Here's how the part is built. I have some questions about the finished solid (model axes, mm). Face numbers are marked on the shaded views. Round coordinates to 2 decimals unless told otherwise and drop trailing zeros. Loops run counter-clockwise (first coordinate to the right, second up) from the corner with the lowest first, then second, coordinate; pieces in that order, holes last. Notation, with made-up numbers: M 69.25,72 L 78.25,72 A7 ccw 78.25,78 Z; hole C -37.5,-38.5 d9. An arc over 180 degrees is marked long. Use a Markdown table: item, result.
```python
from build123d import *

# Parameters (mm, degrees)
BOSS_EXTRUDE1_DEPTH = 6
CUT_EXTRUDE1_DEPTH  = 4.5
CUT_EXTRUDE2_DEPTH  = 1.5
FILLET1_R           = 1.5
SKETCH4_W           = 0.6
SKETCH4_H           = 40
SKETCH4_W_2         = 55
SKETCH4_H_2         = 0.6
CUT_EXTRUDE3_DEPTH  = 2.5


with BuildPart() as part:
    # Sketch1 → Boss-Extrude1 (new body)
    with BuildSketch(Plane(origin=(0, 0, 0), x_dir=(1, 0, 0), z_dir=(0, 1, 0))):
        with BuildLine():
            Line((3, 0), (64.1, 0))
            ThreePointArc((64.1, 0), (66.221320344, 0.878679656), (67.1, 3))
            Line((67.1, 3), (67.1, 49))
            ThreePointArc((67.1, 49), (66.221320344, 51.121320344), (64.1, 52))
            Line((64.1, 52), (3, 52))
            ThreePointArc((3, 52), (0.878679656, 51.121320344), (0, 49))
            Line((0, 49), (0, 3))
            ThreePointArc((0, 3), (0.878679656, 0.878679656), (3, 0))
        make_face()
    extrude(amount=BOSS_EXTRUDE1_DEPTH)

    # Sketch2 → Cut-Extrude1 (cut)
    with BuildSketch(Plane(origin=(0, 0, 0), x_dir=(-1, 0, 0), z_dir=(0, -1, 0))):
        with BuildLine():
            Line((-4.9, 1.9), (-62.2, 1.9))
            ThreePointArc((-62.2, 1.9), (-64.321320344, 2.778679656), (-65.2, 4.9))
            Line((-65.2, 4.9), (-65.2, 48.1))
            ThreePointArc((-65.2, 48.1), (-64.321320344, 50.221320344), (-62.2, 51.1))
            Line((-62.2, 51.1), (-4.9, 51.1))
            ThreePointArc((-4.9, 51.1), (-2.778679656, 50.221320344), (-1.9, 48.1))
            Line((-1.9, 48.1), (-1.9, 4.9))
            ThreePointArc((-1.9, 4.9), (-2.778679656, 2.778679656), (-4.9, 1.9))
        make_face()
    extrude(amount=-CUT_EXTRUDE1_DEPTH, mode=Mode.SUBTRACT)

    # Sketch3 → Cut-Extrude2 (cut)
    with BuildSketch(Plane(origin=(0, 6, 0), x_dir=(1, 0, 0), z_dir=(0, 1, 0))):
        with BuildLine():
            Line((26.225, 41.43), (40.475, 41.43))
            ThreePointArc((40.475, 41.43), (41.005330086, 41.210330086), (41.225, 40.68))
            Line((41.225, 40.68), (41.225, 26.43))
            ThreePointArc((41.225, 26.43), (41.005330086, 25.899669914), (40.475, 25.68))
            Line((40.475, 25.68), (26.225, 25.68))
            ThreePointArc((26.225, 25.68), (25.694669914, 25.899669914), (25.475, 26.43))
            Line((25.475, 26.43), (25.475, 40.68))
            ThreePointArc((25.475, 40.68), (25.694669914, 41.210330086), (26.225, 41.43))
        make_face()
        with BuildLine():
            Line((7.175, 22.38), (21.425, 22.38))
            ThreePointArc((21.425, 22.38), (21.955330086, 22.160330086), (22.175, 21.63))
            Line((22.175, 21.63), (22.175, 7.38))
            ThreePointArc((22.175, 7.38), (21.955330086, 6.849669914), (21.425, 6.63))
            Line((21.425, 6.63), (7.175, 6.63))
            ThreePointArc((7.175, 6.63), (6.644669914, 6.849669914), (6.425, 7.38))
            Line((6.425, 7.38), (6.425, 21.63))
            ThreePointArc((6.425, 21.63), (6.644669914, 22.160330086), (7.175, 22.38))
        make_face()
        with BuildLine():
            Line((26.225, 22.38), (40.475, 22.38))
            ThreePointArc((40.475, 22.38), (41.005330086, 22.160330086), (41.225, 21.63))
            Line((41.225, 21.63), (41.225, 7.38))
            ThreePointArc((41.225, 7.38), (41.005330086, 6.849669914), (40.475, 6.63))
            Line((40.475, 6.63), (26.225, 6.63))
            ThreePointArc((26.225, 6.63), (25.694669914, 6.849669914), (25.475, 7.38))
            Line((25.475, 7.38), (25.475, 21.63))
            ThreePointArc((25.475, 21.63), (25.694669914, 22.160330086), (26.225, 22.38))
        make_face()
        with BuildLine():
            Line((45.275, 22.38), (59.525, 22.38))
            ThreePointArc((59.525, 22.38), (60.055330086, 22.160330086), (60.275, 21.63))
            Line((60.275, 21.63), (60.275, 7.38))
            ThreePointArc((60.275, 7.38), (60.055330086, 6.849669914), (59.525, 6.63))
            Line((59.525, 6.63), (45.275, 6.63))
            ThreePointArc((45.275, 6.63), (44.744669914, 6.849669914), (44.525, 7.38))
            Line((44.525, 7.38), (44.525, 21.63))
            ThreePointArc((44.525, 21.63), (44.744669914, 22.160330086), (45.275, 22.38))
        make_face()
    extrude(amount=-CUT_EXTRUDE2_DEPTH, mode=Mode.SUBTRACT)

    # Fillet1
    fillet1_edges = [part.edges().sort_by_distance(p)[0] for p in [
        (66.221320344, 6, -0.878679656),
        (67.1, 6, -26),
        (66.221320344, 6, -51.121320344),
        (33.55, 6, -52),
        (0.878679656, 6, -51.121320344),
        (0, 6, -26),
        (0.878679656, 6, -0.878679656),
        (33.55, 6, 0),
    ]]
    fillet(fillet1_edges, radius=FILLET1_R)

    # Sketch4 → Cut-Extrude3 (cut)
    with BuildSketch(Plane.XZ):
        with Locations((1, -26)):
            Rectangle(SKETCH4_W, SKETCH4_H)
        with Locations((33.55, -1)):
            Rectangle(SKETCH4_W_2, SKETCH4_H_2)
        with Locations((66.1, -26)):
            Rectangle(SKETCH4_W, SKETCH4_H)
    extrude(amount=-CUT_EXTRUDE3_DEPTH, mode=Mode.SUBTRACT)


solid = part.part
```
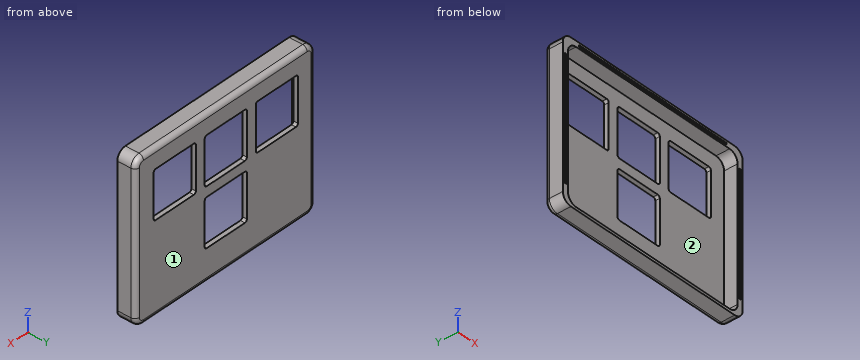
Q1. Imagine slicing it at C-C, the plane z = -9. Give the number of separate pieces and of enclosed holes in the cut face, then the cut area to 3 significant figures.
Return value:
| item | result |
|---|---|
| separate pieces | 4 |
| enclosed holes | 0 |
| area | 42.9 mm^2 |
Q2. I need wall thicknesses on line 1 (X direction, y = 1.8, z = -12); line 2 (Z direction, x = 55.5, y = 2); line 3 (X direction, y = 4.1, z = -7.5). Which ranges of each line are inside material? Lowest first, please. Write a range as from..to.
Return value:
| item | result |
|---|---|
| line 1 | x = 0..0.7, 1.3..1.9, 65.2..65.8, 66.4..67.1 |
| line 2 | z = -52..-51.1, -1.9..-1.3, -0.7..0 |
| line 3 | x = 0..1.9, 65.2..67.1 |
Q3. Imagine slicing it at A-A, the plane z = -32. Please give me the cut outline in (x, y) (3 decimals).
Return value:
| item | result |
|---|---|
| outline | M 0,0 L 0.7,0 L 0.7,2.5 L 1.3,2.5 L 1.3,0 L 1.9,0 L 1.9,4.5 L 25.475,4.5 L 25.475,6 L 1.5,6 A1.5 ccw 0,4.5 Z; M 41.225,4.5 L 65.2,4.5 L 65.2,0 L 65.8,0 L 65.8,2.5 L 66.4,2.5 L 66.4,0 L 67.1,0 L 67.1,4.5 A1.5 ccw 65.6,6 L 41.225,6 Z |
Q4. Imagine slicing it at B-B, the plane x = 54. Please give me the cut outline in (y, z), then the cut area to 3 significant figures.
Return value:
| item | result |
|---|---|
| outline | M 0,-52 L 4.5,-52 A1.5 ccw 6,-50.5 L 6,-22.38 L 4.5,-22.38 L 4.5,-51.1 L 0,-51.1 Z; M 0,-1.9 L 4.5,-1.9 L 4.5,-6.63 L 6,-6.63 L 6,-1.5 A1.5 ccw 4.5,0 L 0,0 L 0,-0.7 L 2.5,-0.7 L 2.5,-1.3 L 0,-1.3 Z |
| area | 64.5 mm^2 |
Q5. We'd pull the mould along Z, two halves only. Please class the marked faces 1 and 2: pulls with the +Z half, pulls with the -Z half, needs draft (parallel to the pull), parting line crosses it, or undercut.
Return value:
| item | result |
|---|---|
| face 1 | needs draft |
| face 2 | undercut |
Q6. Imagine slicing it at D-D, the plane y = 0.9. Please give me the cut outline in (x, z), then the cut area to 3 significant figures.
Return value:
| item | result |
|---|---|
| outline | M 0,-49 A3 ccw 3,-52 L 64.1,-52 A3 ccw 67.1,-49 L 67.1,-3 A3 ccw 64.1,0 L 3,0 A3 ccw 0,-3 Z; hole M 0.7,-46 L 1.3,-46 L 1.3,-6 L 0.7,-6 Z; hole M 1.9,-48.1 A3 ccw 4.9,-51.1 L 62.2,-51.1 A3 ccw 65.2,-48.1 L 65.2,-4.9 A3 ccw 62.2,-1.9 L 4.9,-1.9 A3 ccw 1.9,-4.9 Z; hole M 6.05,-1.3 L 61.05,-1.3 L 61.05,-0.7 L 6.05,-0.7 Z; hole M 65.8,-46 L 66.4,-46 L 66.4,-6 L 65.8,-6 Z |
| area | 294 mm^2 |
Q7. Will these pins go through, and if not, where does the flat tip stop? P1, Ø0.7, axis at x = 46, z = -1, coming from the -Y side; P2, Ø0.8, axis at y = 5.5, z = -16.5, coming from the +X side.
Return value:
| item | result |
|---|---|
| P1 | stops at y = 0 |
| P2 | stops at x = 66.97 |
